Verification items for the finished model (mm, model axes). Face numbers are marked on the shaded views. Round coordinates to 2 decimals unless told otherwise and drop trailing zeros. Write each loop counter-clockwise with the first axis right and the second up, starting at its lowest first coordinate (ties: lowest second). Pieces come first, ordered by that corner, then holes. Notation, with made-up numbers: M -3.75,24 L 45.25,24 A31 cw 45.25,50 Z; hole C 38,44.25 d7. An arc over 180 degrees is marked long. One line per question, with ' | ' between items. Start each with the question number.
Q1. Cross-section at A-A (x = 0). Record the boundary of the cut face in (y, z), then the cut area to 3 significant figures.
Q2. Cross-section at D-D (y = 8.75). Record the boundary of the cut face in (x, z).
Q3. Gauge pin test, flat ends, axial feed: pin 1 (1 mm diameter, centred on y = 6, z = 1, fed in from +X); pin 2 (4 mm diameter, centred on y = 5.5, z = 3, fed in from +X); pin 3 (4 mm diameter, centred on x = -2, z = 1.5, fed in from -Y); pin 4 (5 mm diameter, centred on x = 4.5, y = 1.5, fed in from -Z). Record the tip position at first contact, or that the pin passes through.
Q4. Release check for a two-part mould opening along Z. For the marked faces 1, 2 and 3 record: released by +Z, released by -Z, zero draft, split by the parting line, or undercut.
Q5. Cross-section at B-B (z = 0). Record the boundary of the cut face in (x, y).
Q6. Thickness scan on line 1 along X through (y, z) = (1, 1.75); line 2 along X through (y, z) = (4.75, -0.75); line 3 along Y through (x, z) = (2.25, 2.5). Record the ranges inside material, lowest first. Write a range as from..to.
Q7. Cross-section at C-C (y = 3.5). Record the boundary of the cut face in (x, z), then the cut area to 3 significant figures.
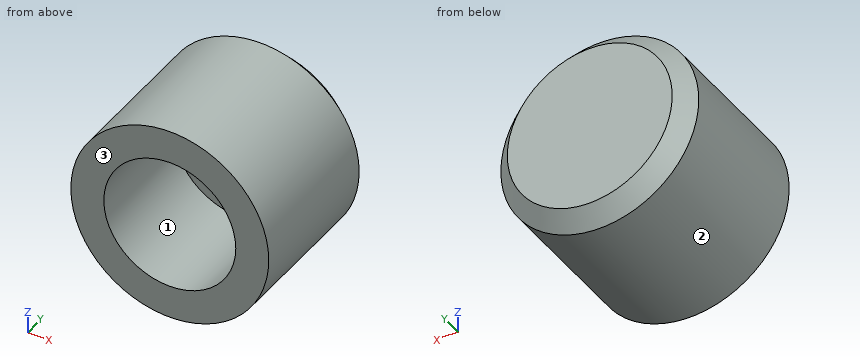
from build123d import *

# Parameters (mm, degrees)
SKETCH1_R           = 6
BOSS_EXTRUDE1_DEPTH = 10
CHAMFER1_SIZE       = 1
SKETCH2_R           = 4
CUT_EXTRUDE1_DEPTH  = 7


with BuildPart() as part:
    # Sketch1 → Boss-Extrude1 (new body)
    with BuildSketch(Plane(origin=(0, 0, 0), x_dir=(1, 0, 0), z_dir=(0, 1, 0))):
        Circle(SKETCH1_R)
    extrude(amount=BOSS_EXTRUDE1_DEPTH)

    # Chamfer1
    chamfer1_edges = [part.edges().sort_by_distance(p)[0] for p in [
        (-6, 10, 0),
    ]]
    chamfer(chamfer1_edges, length=CHAMFER1_SIZE)

    # Sketch2 → Cut-Extrude1 (cut)
    with BuildSketch(Plane.XZ):
        Circle(SKETCH2_R)
    extrude(amount=-CUT_EXTRUDE1_DEPTH, mode=Mode.SUBTRACT)


solid = part.part
Determined:
1) outline: M 0,-6 L 9,-6 L 10,-5 L 10,5 L 9,6 L 0,6 L 0,4 L 7,4 L 7,-4 L 0,-4 Z | area: 63.0 mm²
2) outline: C 0,0 d12
3) pin 1: stops at x = 5.98 | pin 2: stops at x = 5.92 | pin 3: stops at y = 0 | pin 4: stops at z = -5.66
4) face 1: undercut | face 2: split by the parting line | face 3: zero draft
5) outline: M -6,0 L -4,0 L -4,7 L 4,7 L 4,0 L 6,0 L 6,9 L 5,10 L -5,10 L -6,9 Z
6) line 1: x = -5.74..-3.6, 3.6..5.74 | line 2: x = -5.95..-3.93, 3.93..5.95 | line 3: y = 7..10
7) outline: C 0,0 d12; hole C 0,0 d8 | area: 62.8 mm²
